Part model, mm, in its own coordinate system. A direction names the side the tool comes from. Give positions to 0.01 mm unless a question says otherwise; leave off trailing zeros. Order: outer loops, then holes, each group sorted by start corner. A loop starts at its lowest first (then second) coordinate and runs counter-clockwise, first axis right, second up. Notation, with made-up numbers: (7.25, 1) - (38.25, 1) arc R27 cw to (38.25, 34) - close; hole circle Ø4 at (-6.75, 0.5). An arc over 180 degrees is marked (long way). One line per item, written item: value.
```python
from build123d import *

# Parameters (mm, degrees)
SKETCH1_R                = 8
SKETCH1_R_2              = 5
BOSS_EXTRUDE1_DEPTH      = 8
WRAP2_SECTION_W          = 4
WRAP2_SECTION_H          = 1
WRAP2_ANGLE              = 57.295779513
WRAP2_SECTOR_2_SECTION_W = 4
WRAP2_SECTOR_2_SECTION_H = 1
WRAP2_SECTOR_2_ANGLE     = 57.295779513
WRAP2_SECTOR_3_SECTION_W = 4
WRAP2_SECTOR_3_SECTION_H = 4
WRAP2_SECTOR_3_ANGLE     = 21.485917317
WRAP2_SECTOR_4_SECTION_W = 4
WRAP2_SECTOR_4_SECTION_H = 4
WRAP2_SECTOR_4_ANGLE     = 21.485917317


with BuildPart() as part:
    # Sketch1 → Boss-Extrude1 (new body)
    with BuildSketch(Plane.XY):
        Circle(SKETCH1_R)
        Circle(SKETCH1_R_2, mode=Mode.SUBTRACT)
    extrude(amount=BOSS_EXTRUDE1_DEPTH)

    # Wrap2 section (on wrap section) → Wrap2 (revolve, cut)
    with BuildSketch(Plane(origin=(0, 0, 0), x_dir=(-0.6416078703161084, -0.7670328159527646, 0), z_dir=(0.7670328159527646, -0.6416078703161084, 0))):
        with Locations((6, -7.5)):
            Rectangle(WRAP2_SECTION_W, WRAP2_SECTION_H)
    revolve(axis=Axis((0, 0, 0), (0, 0, -1)), revolution_arc=WRAP2_ANGLE, mode=Mode.SUBTRACT)

    # Wrap2 sector 2 section (on wrap section) → Wrap2 sector 2 (revolve, cut)
    with BuildSketch(Plane(origin=(0, 0, 0), x_dir=(0.6403854395311468, 0.7680537017920687, 0), z_dir=(-0.7680537017920687, 0.6403854395311468, 0))):
        with Locations((6, -7.5)):
            Rectangle(WRAP2_SECTOR_2_SECTION_W, WRAP2_SECTOR_2_SECTION_H)
    revolve(axis=Axis((0, 0, 0), (0, 0, -1)), revolution_arc=WRAP2_SECTOR_2_ANGLE, mode=Mode.SUBTRACT)

    # Wrap2 sector 3 section (on wrap section) → Wrap2 sector 3 (revolve, cut)
    with BuildSketch(Plane(origin=(0, 0, 0), x_dir=(-0.9691091288804563, -0.24663230996883403, 0), z_dir=(0.24663230996883403, -0.9691091288804563, 0))):
        with Locations((6, -5)):
            Rectangle(WRAP2_SECTOR_3_SECTION_W, WRAP2_SECTOR_3_SECTION_H)
    revolve(axis=Axis((0, 0, 0), (0, 0, -1)), revolution_arc=WRAP2_SECTOR_3_ANGLE, mode=Mode.SUBTRACT)

    # Wrap2 sector 4 section (on wrap section) → Wrap2 sector 4 (revolve, cut)
    with BuildSketch(Plane(origin=(0, 0, 0), x_dir=(0.9687151001182653, 0.24817545165237268, 0), z_dir=(-0.24817545165237268, 0.9687151001182653, 0))):
        with Locations((6, -5)):
            Rectangle(WRAP2_SECTOR_4_SECTION_W, WRAP2_SECTOR_4_SECTION_H)
    revolve(axis=Axis((0, 0, 0), (0, 0, -1)), revolution_arc=WRAP2_SECTOR_4_ANGLE, mode=Mode.SUBTRACT)


solid = part.part
```
1) Which spindle directions (+Z, -Z, +X, -X, +Y, -Y) get a long thin tool onto all of the face, cutting with end or side? Do faces 1 (the face through (-4.157, -4.97, 7.493)), 2 (the face through (3, -5, 8)), 3 (the face through (6.28, 1.61, 4.97)). Say none if no direction does.
Answer:
face 1: +Z, -X
face 2: +Z, +X, -X, +Y, -Y
face 3: +Z, +X
2) Drop flat-ended pins along their axis: P1, Ø1, axis at x = 3.5, y = 2, coming from the +Z side; P2, Ø0.9, axis at x = 6, y = 0, coming from the +Z side; P3, Ø1, axis at y = -4.5, z = 2.5, coming from the +X side; P4, Ø3.5, axis at x = -6.5, y = -4.5, coming from the +Z side. Give the stop position or say it passes through.
Answer:
P1: passes through
P2: stops at z = 3
P3: stops at x = 6.93
P4: stops at z = 7
3) Slice it at D-D on z = 2.25. Write the cut outline in (x, y).
Answer:
outline: circle Ø16 at (0, 0); hole circle Ø10 at (0, 0)
4) Two-plate mould, pull along Y, no slides. Class faces 4 (the face through (4.77, 1.5, 3.94)), 5 (the face through (7.63, 2.4, 3.94)), 6 (the face through (4.15, 4.98, 7.49)), 7 (the face through (5.2, 0.1, 0)): pulls with the +Y half, pulls with the -Y half, needs draft (parallel to the pull), parting line crosses it, or undercut.
Answer:
face 4: undercut
face 5: parting line crosses it
face 6: undercut
face 7: needs draft
5) Slice it at B-B on x = 0. Write the cut outline in (y, z).
Answer:
outline: (-8, 0) - (-5, 0) - (-5, 8) - (-8, 8) - close; (5, 0) - (8, 0) - (8, 8) - (5, 8) - close
6) Wall check: line 1 along Y through (x, z) = (0, 1.75); line 2 along X through (y, z) = (2.5, 0.5). Give the ranges that are in metal, low to high. Write a range as [from, to].
Answer:
line 1: y = [-8, -5], [5, 8]
line 2: x = [-7.6, -4.33], [4.33, 7.6]
7) Slice it at A-A on z = 7.25. Write the cut outline in (x, y), then the cut area to 3 significant figures.
Answer:
outline: (-7.94, 1) - (-4.96, 0.63) arc R5 cw to (3.2, 3.84) - (5.12, 6.14) arc R8 ccw to start; (-5.13, -6.14) arc R8 ccw to (7.94, -0.99) - (4.96, -0.62) arc R5 cw to (-3.21, -3.84) - close
area: 83.5 mm2
8) Slice it at C-C on y = -1.5. Write the cut outline in (x, z).
Answer:
outline: (-7.86, 0) - (-4.77, 0) - (-4.77, 7) - (-5.89, 7) - (-5.89, 3) - (-7.86, 3) - close; (4.77, 0) - (7.86, 0) - (7.86, 8) - (4.77, 8) - close
